from build123d import *

# Parameters (mm, degrees)
F0_W      = 19
F0_H      = 12
F1_DEPTH  = 6
F3_DEPTH  = 4.2
F2_W      = 19
F2_H      = 2.1
F4_DEPTH  = 3
F6_DEPTH  = 19
F7_R      = 2
F8_W      = 6.1
F8_H      = 1
F9_DEPTH  = 0.8
F11_DEPTH = 4.5


with BuildPart() as f1:
    # F0 (on Front) → F1 (new body)
    with BuildSketch(Plane.XZ):
        Rectangle(F0_W, F0_H)
    extrude(amount=F1_DEPTH)

    # F2 (on face) → F3 (cut)
    with BuildSketch(Plane.XZ.offset(6)):
        with BuildLine():
            ThreePointArc((6.25, -0.4), (5.312742, 1.862742), (3.05, 2.8))
            Line((3.05, 2.8), (-3.05, 2.8))
            ThreePointArc((-3.05, 2.8), (-5.312742, 1.862742), (-6.25, -0.4))
            Line((-6.25, -0.4), (-6.25, -1.55))
            ThreePointArc((-6.25, -1.55), (-5.312742, -3.812742), (-3.05, -4.75))
            Line((-3.05, -4.75), (3.05, -4.75))
            ThreePointArc((3.05, -4.75), (5.312742, -3.812742), (6.25, -1.55))
            Line((6.25, -1.55), (6.25, -0.4))
        make_face()
    extrude(amount=-F3_DEPTH, mode=Mode.SUBTRACT)

    # F2 (on face) → F4 (cut)
    with BuildSketch(Plane.XZ.offset(6)):
        with Locations((0, 4.95)):
            Rectangle(F2_W, F2_H)
    extrude(amount=-F4_DEPTH, mode=Mode.SUBTRACT)

    # F5 (on face) → F6 (join, through all)
    with BuildSketch(Plane.YZ.offset(9.5)):
        Polygon((-3, 5.3), (-3, 6), (-6, 6), (-6, 5.3), (-4.5, 5.3), align=None)
        Polygon((-4.5, 5.3), (-6, 5.3), (-6, 4.60372), align=None)
    extrude(amount=-F6_DEPTH)

    # F7
    f7_edges = [f1.edges().sort_by_distance(p)[0] for p in [
        (0, 0, 6),
        (0, 0, -6),
    ]]
    fillet(f7_edges, radius=F7_R)

    # F8 (on face) → F9 (cut)
    with BuildSketch(Plane.XY.offset(-4.75)):
        with Locations((0, -4.594713)):
            Rectangle(F8_W, F8_H)
    extrude(amount=-F9_DEPTH, mode=Mode.SUBTRACT)

    # F10 (on face) → F11 (join)
    with BuildSketch(Plane.XZ.offset(1.8)):
        with BuildLine():
            Line((-5.25, -0.4), (-5.25, -1.55))
            ThreePointArc((-5.25, -1.55), (-4.605635, -3.105635), (-3.05, -3.75))
            Line((-3.05, -3.75), (3.05, -3.75))
            ThreePointArc((3.05, -3.75), (4.605635, -3.105635), (5.25, -1.55))
            Line((5.25, -1.55), (5.25, -0.4))
            ThreePointArc((5.25, -0.4), (4.605635, 1.155635), (3.05, 1.8))
            Line((3.05, 1.8), (-3.05, 1.8))
            ThreePointArc((-3.05, 1.8), (-4.605635, 1.155635), (-5.25, -0.4))
        make_face()
    extrude(amount=F11_DEPTH)


solid = f1.part
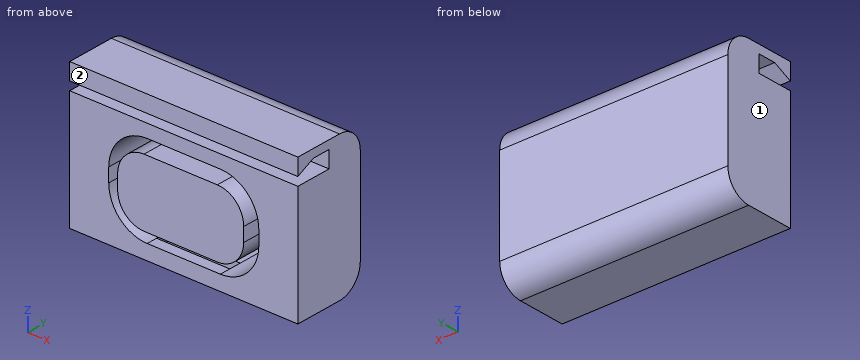
Geometry: final body of the model. Coordinates: model frame, mm. Face numbers are marked on the shaded views. A direction names the side the tool comes from. Round coordinates to 2 decimals unless told otherwise and drop trailing zeros. Order: outer loops, then holes, each group sorted by start corner. A loop starts at its lowest first (then second) coordinate and runs counter-clockwise, first axis right, second up.
Q1. Section C-C, the plane x = 6. Output: boundary loops of the cut face in (y, z), and give its area (3 significant figures).
Result sheet:
outline: (-6, -6) - (-2, -6) arc R2 ccw to (0, -4) - (0, 4) arc R2 ccw to (-2, 6) - (-6, 6) - (-6, 4.6) - (-4.5, 5.3) - (-3, 5.3) - (-3, 3.9) - (-6, 3.9) - (-6, 0.84) - (-1.8, 0.84) - (-1.8, -2.79) - (-6, -2.79) - close
area: 51.4 mm2
Q2. Material intervals for probe 1 along X at (y, z) = (-3.75, -0.25); probe 2 along Z at (x, y) = (-1.5, -2.25); probe 3 along X at (y, z) = (-4.25, 1.5), sorted ascending.
Result sheet:
probe 1: x = -9.5 to -6.25, -5.24 to 5.24, 6.25 to 9.5
probe 2: z = -6 to -4.75, -3.75 to 1.8, 2.8 to 6
probe 3: x = -9.5 to -5.62, -4.16 to 4.16, 5.62 to 9.5
Q3. Section D-D, the plane x = 2.75. Output: boundary loops of the cut face in (y, z), and give its area (3 significant figures).
Result sheet:
outline: (-6.3, -3.75) - (-1.8, -3.75) - (-1.8, -4.75) - (-4.09, -4.75) - (-4.09, -5.55) - (-5.09, -5.55) - (-5.09, -4.75) - (-6, -4.75) - (-6, -6) - (-2, -6) arc R2 ccw to (0, -4) - (0, 4) arc R2 ccw to (-2, 6) - (-6, 6) - (-6, 4.6) - (-4.5, 5.3) - (-3, 5.3) - (-3, 3.9) - (-6, 3.9) - (-6, 2.8) - (-1.8, 2.8) - (-1.8, 1.8) - (-6.3, 1.8) - close
area: 59.1 mm2
Q4. Section B-B, the plane z = -1. Output: boundary loops of the cut face in (x, y).
Result sheet:
outline: (-9.5, -6) - (-6.25, -6) - (-6.25, -1.8) - (-5.25, -1.8) - (-5.25, -6.3) - (5.25, -6.3) - (5.25, -1.8) - (6.25, -1.8) - (6.25, -6) - (9.5, -6) - (9.5, 0) - (-9.5, 0) - close
Q5. Access query for the marked faces 1 and 2. Directions: +Z, -Z, +X, -X, +Y, -Y. A direction counts if a zero-diameter tool reaches every point of the face in a straight line with its end or side. Return the directions, or none.
Result sheet:
face 1: +Z, -Z, -X, +Y, -Y
face 2: +Z, +X, -X, -Y
Q6. Section A-A, the plane y = -3.5. Output: boundary loops of the cut face in (x, z).
Result sheet:
outline: (-9.5, -6) - (9.5, -6) - (9.5, 3.9) - (-9.5, 3.9) - close; (-9.5, 5.3) - (9.5, 5.3) - (9.5, 6) - (-9.5, 6) - close; (-5.25, -1.55) arc R2.2 ccw to (-3.05, -3.75) - (3.05, -3.75) arc R2.2 ccw to (5.25, -1.55) - (5.25, -0.4) arc R2.2 ccw to (3.05, 1.8) - (-3.05, 1.8) arc R2.2 ccw to (-5.25, -0.4) - close; hole (-6.25, -1.55) arc R3.2 ccw to (-3.05, -4.75) - (3.05, -4.75) arc R3.2 ccw to (6.25, -1.55) - (6.25, -0.4) arc R3.2 ccw to (3.05, 2.8) - (-3.05, 2.8) arc R3.2 ccw to (-6.25, -0.4) - close
